```python
from build123d import *

# Parameters (mm, degrees)
MODEL_R             = 0.5842
MODEL_R_2           = 1.5748
BOSS_EXTRUDE1_DEPTH = 1.5748
SKETCH1_R           = 2.4257
BOSS_EXTRUDE2_DEPTH = 1.27
SKETCH2_R           = 1.905
BOSS_EXTRUDE3_DEPTH = 2.8956
SKETCH3_R           = 1.7526
BOSS_EXTRUDE4_DEPTH = 7.8486
SKETCH4_R           = 1.143
BOSS_EXTRUDE5_DEPTH = 10.0838
SKETCH5_R           = 0.508
BOSS_EXTRUDE6_DEPTH = 2.794


with BuildPart() as part:
    # Model → Boss-Extrude1 (new body)
    with BuildSketch(Plane.XY):
        Polygon((0, 11.43), (1.27, 12.7), (26.67, 12.7), (27.94, 11.43), (27.94, 1.27), (26.67, 0), (1.27, 0), (0, 1.27), align=None)
        with Locations((10.795, 6.35)):
            Circle(MODEL_R, mode=Mode.SUBTRACT)
        with Locations((17.145, 6.35)):
            Circle(MODEL_R, mode=Mode.SUBTRACT)
        with Locations((3.81, 6.35)):
            Circle(MODEL_R_2, mode=Mode.SUBTRACT)
        with Locations((24.13, 6.35)):
            Circle(MODEL_R_2, mode=Mode.SUBTRACT)
        with Locations((13.335, 3.175)):
            Circle(MODEL_R, mode=Mode.SUBTRACT)
        with Locations((14.605, 9.525)):
            Circle(MODEL_R, mode=Mode.SUBTRACT)
    extrude(amount=BOSS_EXTRUDE1_DEPTH)

    # Sketch1 → Boss-Extrude2 (add)
    with BuildSketch(Plane.XY.offset(1.5748)):
        with Locations(Location((10.795, 6.35, 0), (0, 0, 180))):
            Circle(SKETCH1_R)
        with Locations(Location((17.145, 6.35, 0), (0, 0, 180))):
            Circle(SKETCH1_R)
    extrude(amount=BOSS_EXTRUDE2_DEPTH)

    # Sketch2 → Boss-Extrude3 (add)
    with BuildSketch(Plane.XY.offset(1.5748)):
        with Locations((10.795, 6.35)):
            Circle(SKETCH2_R)
        with Locations((17.145, 6.35)):
            Circle(SKETCH2_R)
    extrude(amount=BOSS_EXTRUDE3_DEPTH)

    # Sketch3 → Boss-Extrude4 (add)
    with BuildSketch(Plane.XY.offset(1.5748)):
        with Locations((17.145, 6.35)):
            Circle(SKETCH3_R)
        with Locations((10.795, 6.35)):
            Circle(SKETCH3_R)
    extrude(amount=BOSS_EXTRUDE4_DEPTH)

    # Sketch4 → Boss-Extrude5 (add)
    with BuildSketch(Plane.XY.offset(1.5748)):
        with Locations((17.145, 6.35)):
            Circle(SKETCH4_R)
        with Locations((10.795, 6.35)):
            Circle(SKETCH4_R)
    extrude(amount=BOSS_EXTRUDE5_DEPTH)

    # Sketch5 → Boss-Extrude6 (add)
    with BuildSketch(Plane(origin=(0, 0, 1.5748), x_dir=(-1, 0, 0), z_dir=(0, 0, -1))):
        with Locations(Location((-17.145, 6.35, 0), (0, 0, 180))):
            Circle(SKETCH5_R)
        with Locations(Location((-10.795, 6.35, 0), (0, 0, 180))):
            Circle(SKETCH5_R)
    extrude(amount=BOSS_EXTRUDE6_DEPTH)


solid = part.part
```
Part model, mm, in its own coordinate system. A direction names the side the tool comes from. Coordinates: 2 decimals unless noted, no trailing zeros. Order: outer loops, then holes, each group sorted by start corner. A loop starts at its lowest first (then second) coordinate and runs counter-clockwise, first axis right, second up. Notation, with made-up numbers: (73.25, -7) - (126.25, -7) arc R27 cw to (126.25, 29) - close; hole circle Ø8 at (20, 24). An arc over 180 degrees is marked (long way). Return JSON: item names as keys, results as strings. Group by question number.
Item 1: Pin check, flat tips, straight feed: pin 1 (6 mm diameter, centred on x = 15, z = 6.5, fed in from +Y) (3 decimals); pin 2 (1.3 mm diameter, centred on x = 13.335, y = 3.175, fed in from +Z); pin 3 (1 mm diameter, centred on x = 11.5, y = 9, fed in from +Z). Stop position of each tip, or through.
Item 2: Which spindle directions (+Z, -Z, +X, -X, +Y, -Y) get a long thin tool onto all of the face, cutting with end or side? Do faces 4 (the face through (12.612, 6.922, 3.646)), 5 (the face through (17, 6, 11.659)). Say none if no direction does.
Item 3: Cut at C-C (y = 6.35). State how many separate pieces and enclosed holes the cut face has, plus the area to 3 significant figures.
Item 4: Pull direction X, two halves, no side cores. Call faces 1 (the face through (18.905, 5.62, 3.646)), 2 (the face through (27.94, 6, 1)), 3 (the face through (17.1, 6.3, -1.219)): pulls with the +X half, pulls with the -X half, needs draft (parallel to the pull), parting line crosses it, or undercut.
Item 5: Drill centre lines: probe 1 along Y at (x, z) = (3.75, 1.25); probe 2 along Z at (x, y) = (17.25, 10.75); probe 3 along X at (y, z) = (6.5, 10). Where is each one in solid material? Low to high. Write a range as from..to.
Item 6: Cut at A-A (x = 24.13). List the corners of the cut face in (y, z), plus the area to 3 significant figures.
Item 7: Cut at B-B (z = 9.75). List the corners of the cut face in (x, y) (3 decimals), plus the area to 3 significant figures.
Item 8: Cut at D-D (x = 6.5). List the corners of the cut face in (y, z), plus the area to 3 significant figures.
Check values:
{
 "1": {"pin 1": "stops at y = 8.255", "pin 2": "stops at z = 1.57", "pin 3": "stops at z = 2.84"},
 "2": {"face 4": "+Z", "face 5": "+Z, +X, -X, +Y, -Y"},
 "3": {"separate pieces": "3", "enclosed holes": "0", "area": "106 mm2"},
 "4": {"face 1": "undercut", "face 2": "pulls with the +X half", "face 3": "needs draft"},
 "5": {"probe 1": "y = 0..4.78, 7.92..12.7", "probe 2": "z = 0..1.57", "probe 3": "x = 9.66..11.93, 16.01..18.28"},
 "6": {"outline": "(0, 0) - (4.78, 0) - (4.78, 1.57) - (0, 1.57) - close; (7.92, 0) - (12.7, 0) - (12.7, 1.57) - (7.92, 1.57) - close", "area": "15.0 mm2"},
 "7": {"outline": "circle Ø2.286 at (10.795, 6.35); circle Ø2.286 at (17.145, 6.35)", "area": "8.21 mm2"},
 "8": {"outline": "(0, 0) - (12.7, 0) - (12.7, 1.57) - (0, 1.57) - close", "area": "20.0 mm2"}
}
